```python
from build123d import *

# Parameters (mm, degrees)
SKETCH1_W                   = 127
SKETCH1_H                   = 101.6
BOSS_EXTRUDE1_DEPTH         = 2.54
TAP_DRILL_FOR_M3X0_5_TAP1_D = 2.5


with BuildPart() as part:
    # Sketch1 → Boss-Extrude1 (new body)
    with BuildSketch(Plane(origin=(0, 0, 0), x_dir=(1, 0, 0), z_dir=(0, 1, 0))):
        with Locations((63.5, -50.8)):
            Rectangle(SKETCH1_W, SKETCH1_H)
    extrude(amount=BOSS_EXTRUDE1_DEPTH)

    # Tap Drill for M3x0.5 Tap1 (through all)
    with Locations(Plane(origin=(0, 0, 0), x_dir=(-1, 0, 0), z_dir=(0, -1, 0))):
        with Locations((-106, -76.6), (-120, -5), (-120, -25), (-106, -5), (-106, -25), (-120, -76.6), (-131.288, -76.6), (-120, -96.6), (-106, -96.6), (-21, -96.6), (-21, -76.6), (-7.112, -76.6), (-7, -96.6), (-21, -25), (-21, -5), (-7, -5), (-7, -25)):
            Hole(TAP_DRILL_FOR_M3X0_5_TAP1_D / 2)

    # Sketch7 → Loft1 section 0
    with BuildSketch(Plane(origin=(0, 9.398, 0), x_dir=(1, 0, 0), z_dir=(0, 1, 0))):
        with BuildLine():
            Line((82.55, 0), (44.45, 0))
            Line((44.45, 0), (44.45, -101.6))
            Line((44.45, -101.6), (82.55, -101.6))
            Line((82.55, -101.6), (82.55, 0))
        make_face()
    # Sketch6 → Loft1 section 1
    with BuildSketch(Plane(origin=(0, 2.54, 0), x_dir=(1, 0, 0), z_dir=(0, 1, 0))):
        with BuildLine():
            Line((35.56, 0), (91.44, 0))
            Line((91.44, 0), (91.44, -101.6))
            Line((91.44, -101.6), (35.56, -101.6))
            Line((35.56, -101.6), (35.56, 0))
        make_face()
    loft()


solid = part.part
```
Geometry check sheet. Reference: the model listing, model coordinates, mm. A direction names the side the tool comes from. Coordinates: 2 decimals unless noted, no trailing zeros. Write each loop counter-clockwise with the first axis right and the second up, starting at its lowest first coordinate (ties: lowest second). Pieces come first, ordered by that corner, then holes. Notation, with made-up numbers: M -24,-39.75 L 4,-39.75 A10 cw 4,-24.75 Z; hole C -30,34 d3. An arc over 180 degrees is marked long. Answer as a JSON object with one key per item and string values.
1. Draft check along Z on faces 1 (the flat face through (0, 1, 52)), 2 (the cylindrical face through (121.155, 1.288, 5.479)), 3 (the flat face through (63, 4, 101.6)), 4 (the cylindrical face through (21.577, 1.288, 77.709)). Enter one of: released by +Z, released by -Z, zero draft, split by the parting line, or undercut.
Answers below:
{"face 1": "zero draft", "face 2": "undercut", "face 3": "released by +Z", "face 4": "undercut"}
2. Tool access check on faces 5 (the flat face through (63, 9.398, 50)), 6 (the flat face through (109, 2.54, 50)). Record the directions out of +Z, -Z, +X, -X, +Y, -Y that give a thin tool (end or side, any length) a straight path to the whole face; none if there is none.
Answers below:
{"face 5": "+Z, -Z, +X, -X, +Y", "face 6": "+Z, -Z, +X, +Y"}
3. Section check B-B, the plane y = 5.5. Enter the section's corners in (x, z), plus the area to 3 significant figures.
Answers below:
{"outline": "M 39.4,0 L 87.6,0 L 87.6,101.6 L 39.4,101.6 Z", "area": "4,900 mm²"}
4. Scan lines: L1, parallel to Z at x = 21, y = 0.8; L2, parallel to X at y = 1.4, z = 96.6; L3, parallel to X at y = 1.5, z = 77. Record each from-to range of solid material in increasing order.
Answers below:
{"L1": "z = 0 to 3.75, 6.25 to 23.75, 26.25 to 75.35, 77.85 to 95.35, 97.85 to 101.6", "L2": "x = 0 to 5.75, 8.25 to 19.75, 22.25 to 104.75, 107.25 to 118.75, 121.25 to 127", "L3": "x = 0 to 5.93, 8.3 to 19.82, 22.18 to 104.82, 107.18 to 118.82, 121.18 to 127"}
5. Section check C-C, the plane x = 33. Enter the section's corners in (y, z), plus the area to 3 significant figures.
Answers below:
{"outline": "M 0,0 L 2.54,0 L 2.54,101.6 L 0,101.6 Z", "area": "258 mm²"}
6. Go/stop test with flat-tipped pins: pin 1 Ø2 at (x, z) = (7.112, 76.6) entering from +Y; pin 2 Ø3 at (x, z) = (120, 76.6) entering from +Y. Record where each tip stops, or that it passes through.
Answers below:
{"pin 1": "passes through", "pin 2": "stops at y = 2.54"}
7. Section check A-A, the plane z = 89. Enter the section's corners in (x, y), plus the area to 3 significant figures.
Answers below:
{"outline": "M 0,0 L 127,0 L 127,2.54 L 91.44,2.54 L 82.55,9.4 L 44.45,9.4 L 35.56,2.54 L 0,2.54 Z", "area": "645 mm²"}
